Design review of the part built by this model. Coordinates are the model's own, in mm. Face numbers are marked on the shaded views. A direction names the side the tool comes from. Round coordinates to 2 decimals unless told otherwise and drop trailing zeros. Loops run counter-clockwise (first coordinate to the right, second up) from the corner with the lowest first, then second, coordinate; pieces in that order, holes last. Notation, with made-up numbers: (28, 48) - (80, 48) arc R22 cw to (80, 64) - close; hole circle Ø7 at (-21.75, 3.25). An arc over 180 degrees is marked (long way). Return JSON: item names as keys, results as strings. Group by question number.
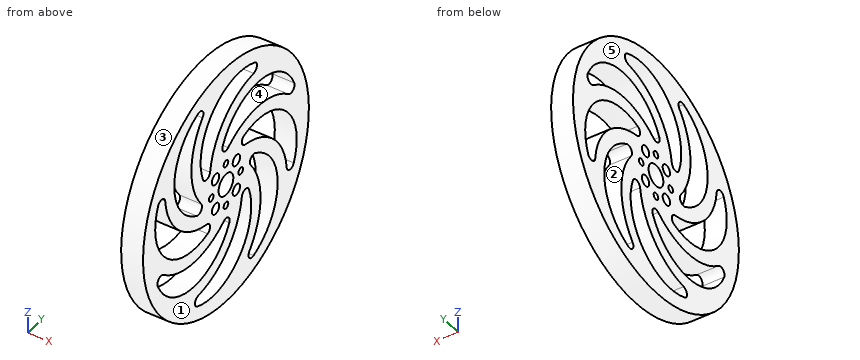
from build123d import *

# Parameters (mm, degrees)
SPROCKET_R                   = 45
ESTRUSIONE_ESTRUSIONE2_DEPTH = 8
SCHIZZO1_R                   = 4
SCHIZZO1_R_2                 = 2
SCHIZZO1_R_3                 = 1.25
TAGLIO_ESTRUSIONE2_DEPTH     = 9
TAGLIO_ESTRUSIONE3_DEPTH     = 9


with BuildPart() as part:
    # Sprocket → Estrusione-Estrusione2 (new body)
    with BuildSketch(Plane(origin=(0, 0, 0), x_dir=(0, 0, -1), z_dir=(1, 0, 0))):
        Circle(SPROCKET_R)
    extrude(amount=ESTRUSIONE_ESTRUSIONE2_DEPTH)

    # Schizzo1 → Taglio-Estrusione2 (cut, through all)
    with BuildSketch(Plane(origin=(0, 0, 0), x_dir=(0, 0, -1), z_dir=(1, 0, 0))):
        Circle(SCHIZZO1_R)
        with Locations((-5.656854249, 5.656854249)):
            Circle(SCHIZZO1_R_2)
        with Locations((5.656854249, 5.656854249)):
            Circle(SCHIZZO1_R_2)
        with Locations((0, 8)):
            Circle(SCHIZZO1_R_3)
        with Locations((8, 0)):
            Circle(SCHIZZO1_R_3)
        with Locations((-8, 0)):
            Circle(SCHIZZO1_R_3)
        with Locations((0, -8)):
            Circle(SCHIZZO1_R_3)
        with Locations((5.656854249, -5.656854249)):
            Circle(SCHIZZO1_R_2)
        with Locations((-5.656854249, -5.656854249)):
            Circle(SCHIZZO1_R_2)
    extrude(amount=TAGLIO_ESTRUSIONE2_DEPTH, mode=Mode.SUBTRACT)

    # Schizzo2 → Taglio-Estrusione3 (cut, through all)
    with BuildSketch(Plane(origin=(8, 0, 0), x_dir=(0, 0, -1), z_dir=(1, 0, 0))):
        with BuildLine():
            ThreePointArc((10.336761524, 8.624888754), (25.791574711, 0.750648199), (32.987627274, -15.031358723))
            ThreePointArc((32.987627274, -15.031358723), (34.683367414, -16.825784979), (36.829895727, -15.605983186))
            ThreePointArc((36.829895727, -15.605983186), (32.508005906, 7.181633564), (9.929440233, 12.488476401))
            ThreePointArc((9.929440233, 12.488476401), (8.617624488, 10.396912474), (10.336761524, 8.624888754))
        make_face()
        with BuildLine():
            ThreePointArc((-1.809511828, 15.851860872), (-1.2581466, 13.445308027), (1.210476844, 13.407911494))
            ThreePointArc((1.210476844, 13.407911494), (17.706608944, 18.768185808), (33.954550624, 12.696999257))
            ThreePointArc((33.954550624, 12.696999257), (36.42247095, 12.627217636), (37.077765557, 15.007572481))
            ThreePointArc((37.077765557, 15.007572481), (17.908449626, 28.064813212), (-1.809511828, 15.851860872))
        make_face()
        with BuildLine():
            ThreePointArc((13.407911494, -1.210476844), (18.768185808, -17.706608944), (12.696999257, -33.954550624))
            ThreePointArc((12.696999257, -33.954550624), (12.627217636, -36.42247095), (15.007572481, -37.077765557))
            ThreePointArc((15.007572481, -37.077765557), (28.064813212, -17.908449626), (15.851860872, 1.809511828))
            ThreePointArc((15.851860872, 1.809511828), (13.445308027, 1.2581466), (13.407911494, -1.210476844))
        make_face()
        with BuildLine():
            ThreePointArc((8.624888754, -10.336761524), (0.750648199, -25.791574711), (-15.031358723, -32.987627274))
            ThreePointArc((-15.031358723, -32.987627274), (-16.825784979, -34.683367414), (-15.605983186, -36.829895727))
            ThreePointArc((-15.605983186, -36.829895727), (7.181633564, -32.508005906), (12.488476401, -9.929440233))
            ThreePointArc((12.488476401, -9.929440233), (10.396912474, -8.617624488), (8.624888754, -10.336761524))
        make_face()
        with BuildLine():
            ThreePointArc((-1.210476844, -13.407911494), (-17.706608944, -18.768185808), (-33.954550624, -12.696999257))
            ThreePointArc((-33.954550624, -12.696999257), (-36.42247095, -12.627217636), (-37.077765557, -15.007572481))
            ThreePointArc((-37.077765557, -15.007572481), (-17.908449626, -28.064813212), (1.809511828, -15.851860872))
            ThreePointArc((1.809511828, -15.851860872), (1.2581466, -13.445308027), (-1.210476844, -13.407911494))
        make_face()
        with BuildLine():
            ThreePointArc((-10.336761524, -8.624888754), (-25.791574711, -0.750648199), (-32.987627274, 15.031358723))
            ThreePointArc((-32.987627274, 15.031358723), (-34.683367414, 16.825784979), (-36.829895727, 15.605983186))
            ThreePointArc((-36.829895727, 15.605983186), (-32.508005906, -7.181633564), (-9.929440233, -12.488476401))
            ThreePointArc((-9.929440233, -12.488476401), (-8.617624488, -10.396912474), (-10.336761524, -8.624888754))
        make_face()
        with BuildLine():
            ThreePointArc((-13.407911494, 1.210476844), (-18.768185808, 17.706608944), (-12.696999257, 33.954550624))
            ThreePointArc((-12.696999257, 33.954550624), (-12.627217636, 36.42247095), (-15.007572481, 37.077765557))
            ThreePointArc((-15.007572481, 37.077765557), (-28.064813212, 17.908449626), (-15.851860872, -1.809511828))
            ThreePointArc((-15.851860872, -1.809511828), (-13.445308027, -1.2581466), (-13.407911494, 1.210476844))
        make_face()
        with BuildLine():
            ThreePointArc((-8.624888754, 10.336761524), (-0.750648199, 25.791574711), (15.031358723, 32.987627274))
            ThreePointArc((15.031358723, 32.987627274), (16.825784979, 34.683367414), (15.605983186, 36.829895727))
            ThreePointArc((15.605983186, 36.829895727), (-7.181633564, 32.508005906), (-12.488476401, 9.929440233))
            ThreePointArc((-12.488476401, 9.929440233), (-10.396912474, 8.617624488), (-8.624888754, 10.336761524))
        make_face()
    extrude(amount=-TAGLIO_ESTRUSIONE3_DEPTH, mode=Mode.SUBTRACT)


solid = part.part
Q1. Draft analysis for pull direction Z (two halves, no side actions). For the marked faces 1, 2 and 3, state which applies: pulls with the +Z half, pulls with the -Z half, needs draft (parallel to the pull), parting line crosses it, or undercut.
Q2. Insertion check: pin 1 Ø3 at (y, z) = (23, 10.5) entering from -X; pin 2 Ø4 at (x, y) = (3.5, 30.5) entering from +Z; pin 3 Ø1.5 at (x, z) = (7, 22) entering from -Y. Each pin has a flat end and moves straight along its axis. Give the tip position at first contact, or say it passes through.
Q3. Add section B-B, the plane z = -21. State the section outline as (x, y) points.
Q4. For line 1 (Y direction, x = 6.5, z = -15); line 2 (Z direction, x = 4, y = 3.5); line 3 (Z direction, x = 1.5, y = -19.5), list the stretches that pass through material, from the lowest coordinate up.
Q5. Add section D-D, the plane y = 26.5. State the section outline as (x, z) points, plus the area to 3 significant figures.
Q6. Add section C-C, the plane z = 0. Give the number of separate pieces and of enclosed holes in the cut face, plus the area to 3 significant figures.
Q7. Add section A-A, the plane z = -30. State the section outline as (x, y) points.
Q8. Tool access review of the marked faces 4 and 5: name each direction out of +Z, -Z, +X, -X, +Y, -Y from which nothing blocks a thin tool from reaching the whole face with its end or side.
Evaluation:
{
 "1": {"face 1": "needs draft", "face 2": "undercut", "face 3": "parting line crosses it"},
 "2": {"pin 1": "through", "pin 2": "z = 34.82", "pin 3": "y = -39.67"},
 "3": {"outline": "(0, -39.8) - (8, -39.8) - (8, -33.29) - (0, -33.29) - close; (0, -1.6) - (8, -1.6) - (8, 4.7) - (0, 4.7) - close; (0, 13.39) - (8, 13.39) - (8, 18.49) - (0, 18.49) - close; (0, 27.77) - (8, 27.77) - (8, 39.8) - (0, 39.8) - close"},
 "4": {"line 1": "-42.43 to -37.08, -30.71 to -3.56, 2 to 7.55, 13.64 to 18.69, 27.93 to 32.98, 37.07 to 42.43", "line 2": "-44.86 to -35.33, -22.71 to -1.94, 1.94 to 14.97, 22.86 to 29.1, 38.03 to 44.86", "line 3": "-40.56 to -27.97, -18.67 to -13.61, -5.59 to 0.38, 34.52 to 40.56"},
 "5": {"outline": "(0, -36.37) - (8, -36.37) - (8, -25.47) - (0, -25.47) - close; (0, -9.42) - (8, -9.42) - (8, -0.02) - (0, -0.02) - close; (0, 11.57) - (8, 11.57) - (8, 17.05) - (0, 17.05) - close; (0, 26.05) - (8, 26.05) - (8, 36.37) - (0, 36.37) - close", "area": "289 mm²"},
 "6": {"separate pieces": "8", "enclosed holes": "0", "area": "351 mm²"},
 "7": {"outline": "(0, -33.54) - (8, -33.54) - (8, -5.06) - (0, -5.06) - close; (0, 9.42) - (8, 9.42) - (8, 15.42) - (0, 15.42) - close; (0, 23.97) - (8, 23.97) - (8, 33.54) - (0, 33.54) - close"},
 "8": {"face 4": "+X, -X", "face 5": "+Z, -Z, -X, +Y, -Y"}
}
